from build123d import *

# Parameters (mm, degrees)
PAD_DEPTH = 1.328


with BuildPart() as part:
    # Sketch → Pad (new body, symmetric)
    with BuildSketch(Plane.YZ):
        with BuildLine():
            Line((-350, 0), (370, 0))
            Line((370, 0), (370, -3))
            ThreePointArc((365.095951, -8.899059), (368.613876, -6.835642), (370, -3))
            Line((365.095951, -8.899059), (229.132925, -34.158821))
            ThreePointArc((220, -35), (224.585791, -34.789261), (229.132925, -34.158821))
            Line((220, -35), (-200, -35))
            ThreePointArc((-209.132925, -34.158821), (-204.585791, -34.789261), (-200, -35))
            Line((-209.132925, -34.158821), (-345.095951, -8.899059))
            ThreePointArc((-350, -3), (-348.613876, -6.835642), (-345.095951, -8.899059))
            Line((-350, -3), (-350, 0))
        make_face()
    extrude(amount=PAD_DEPTH, both=True)


solid = part.part
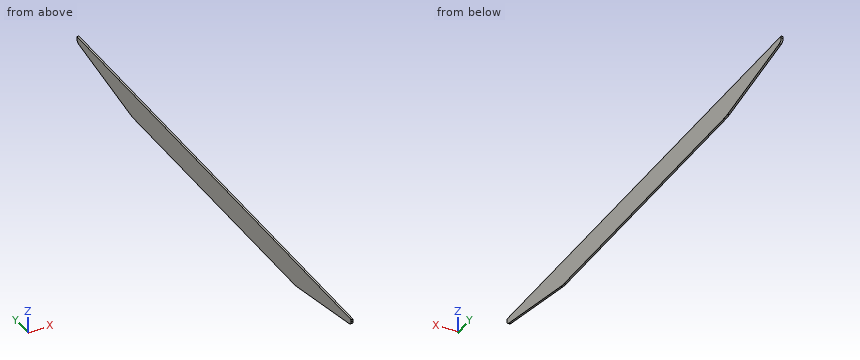
Input: part model. Units: mm. Frame: model coordinates. Give positions to 0.01 mm unless a question says otherwise; leave off trailing zeros. Loops run counter-clockwise (first coordinate to the right, second up) from the corner with the lowest first, then second, coordinate; pieces in that order, holes last. Notation, with made-up numbers: (6, 19.5) -> (32, 19.5) arc R21 cw to (32, 56.5) -> close; hole circle Ø10 at (83.25, -7). An arc over 180 degrees is marked (long way). Answer as a JSON object with one key per item and string values. Group by question number.
Item 1: Cut plane B-B, the plane z = -17. Return the cut outline in (x, y), and give its area (3 significant figures).
Item 2: Cut plane A-A, the plane x = -0.7. Return the cut outline in (y, z), and give its area (3 significant figures).
Item 3: Line query: probe 1 along Z at (x, y) = (-1.2, 241); probe 2 along Z at (x, y) = (-0.1, 248); probe 3 along Y at (x, z) = (0.9, -7.5). Output: solid intervals per line, ascending.
Item 4: Cut plane C-C, the plane y = -286. Return the cut outline in (x, z).
Checks:
{
 "1": {"outline": "(-1.33, -301.49) -> (1.33, -301.49) -> (1.33, 321.49) -> (-1.33, 321.49) -> close", "area": "1,650 mm²"},
 "2": {"outline": "(-350, -3) arc R6 ccw to (-345.1, -8.9) -> (-209.13, -34.16) arc R50 ccw to (-200, -35) -> (220, -35) arc R50 ccw to (229.13, -34.16) -> (365.1, -8.9) arc R6 ccw to (370, -3) -> (370, 0) -> (-350, 0) -> close", "area": "21,300 mm²"},
 "3": {"probe 1": "z = -31.95 to 0", "probe 2": "z = -30.65 to 0", "probe 3": "y = -347.97 to 367.97"},
 "4": {"outline": "(-1.33, -19.88) -> (1.33, -19.88) -> (1.33, 0) -> (-1.33, 0) -> close"}
}
